CAD build for the part. Positions are in the model's coordinates, mm. A direction names the side the tool comes from. Round coordinates to 2 decimals unless told otherwise and drop trailing zeros. Order: outer loops, then holes, each group sorted by start corner. A loop starts at its lowest first (then second) coordinate and runs counter-clockwise, first axis right, second up. Notation, with made-up numbers: M 51,61.25 L 90,61.25 A18 ccw 90,80.25 Z; hole C 77.25,-30 d10. An arc over 180 degrees is marked long. Put each result on its own line as item: value.
```python
from build123d import *

# Parameters (mm, degrees)
BOSS_EXTRUDE1_DEPTH            = 5
SKETCH2_W                      = 135
SKETCH2_H                      = 160
SKETCH2_W_2                    = 125
SKETCH2_H_2                    = 150
BOSS_EXTRUDE2_DEPTH            = 23
SKETCH3_R                      = 4.7
CUT_EXTRUDE1_DEPTH             = 140
SKETCH4_R                      = 4
BOSS_EXTRUDE3_DEPTH            = 47
F_2_5MM_DOWEL_HOLE1_D          = 2.5
F_2_5MM_DOWEL_HOLE1_DEPTH      = 12
F_2_5MM_DOWEL_HOLE1_TIP        = 0.751075774
FILLET1_R                      = 1
SKETCH8_R                      = 2.5
BOSS_EXTRUDE4_DEPTH            = 4
F_2_5_2_5_DIAMETER_HOLE2_D     = 2.5
F_2_5_2_5_DIAMETER_HOLE2_DEPTH = 5
F_2_5_2_5_DIAMETER_HOLE2_TIP   = 0.751075774
FILLET2_R                      = 10


with BuildPart() as part:
    # Sketch1 → Boss-Extrude1 (new body)
    with BuildSketch(Plane(origin=(0, 0, 0), x_dir=(1, 0, 0), z_dir=(0, 1, 0))):
        with BuildLine():
            Line((-67.5, 80), (-67.5, -80))
            Line((-67.5, -80), (67.5, -80))
            Line((67.5, -80), (67.5, 80))
            Line((67.5, 80), (26.490666647, 192.672217375))
            ThreePointArc((26.490666647, 192.672217375), (0, 211.221181853), (-26.490666647, 192.672217375))
            Line((-26.490666647, 192.672217375), (-67.5, 80))
        make_face()
        Polygon((-37.5, 80), (37.5, 80), (0, 183.03040323), align=None, mode=Mode.SUBTRACT)
    extrude(amount=BOSS_EXTRUDE1_DEPTH)

    # Sketch2 → Boss-Extrude2 (add)
    with BuildSketch(Plane(origin=(0, 5, 0), x_dir=(1, 0, 0), z_dir=(0, 1, 0))):
        Rectangle(SKETCH2_W, SKETCH2_H)
        Rectangle(SKETCH2_W_2, SKETCH2_H_2, mode=Mode.SUBTRACT)
    extrude(amount=BOSS_EXTRUDE2_DEPTH)

    # Sketch3 → Cut-Extrude1 (cut)
    with BuildSketch(Plane(origin=(67.5, 0, 0), x_dir=(0, 0, -1), z_dir=(1, 0, 0))):
        with Locations((-45, 28)):
            Circle(SKETCH3_R)
    extrude(amount=-CUT_EXTRUDE1_DEPTH, mode=Mode.SUBTRACT)

    # Sketch4 → Boss-Extrude3 (add)
    with BuildSketch(Plane(origin=(0, 5, 0), x_dir=(1, 0, 0), z_dir=(0, 1, 0))):
        with Locations(Location((-52.5, 65, 0), (0, 0, 90))):
            Circle(SKETCH4_R)
        with Locations(Location((52.5, 65, 0), (0, 0, 90))):
            Circle(SKETCH4_R)
        with Locations(Location((52.5, -65, 0), (0, 0, 90))):
            Circle(SKETCH4_R)
        with Locations(Location((-52.5, -65, 0), (0, 0, 90))):
            Circle(SKETCH4_R)
    extrude(amount=BOSS_EXTRUDE3_DEPTH)

    # Ø2.5mm Dowel Hole1
    with Locations(Plane(origin=(0, 52, 0), x_dir=(1, 0, 0), z_dir=(0, 1, 0))):
        with Locations((-52.5, 65), (52.5, 65), (52.5, -65), (-52.5, -45), (-52.5, -65)):
            Hole(F_2_5MM_DOWEL_HOLE1_D / 2, depth=F_2_5MM_DOWEL_HOLE1_DEPTH)
            with Locations((0, 0, -(F_2_5MM_DOWEL_HOLE1_DEPTH + F_2_5MM_DOWEL_HOLE1_TIP / 2))):  # 118° drill point
                Cone(0, F_2_5MM_DOWEL_HOLE1_D / 2, F_2_5MM_DOWEL_HOLE1_TIP, mode=Mode.SUBTRACT)

    # Fillet1
    fillet1_edges = [part.edges().sort_by_distance(p)[0] for p in [
        (67.5, 14, 80),
        (-67.5, 14, 80),
        (0, 2.5, -183.03040323),
        (0, 0, 80),
        (-67.5, 0, 0),
        (67.5, 0, 0),
    ]]
    fillet(fillet1_edges, radius=FILLET1_R)

    # Sketch8 → Boss-Extrude4 (add)
    with BuildSketch(Plane(origin=(0, 5, 0), x_dir=(1, 0, 0), z_dir=(0, 1, 0))):
        with Locations(Location((-40.82, 15.565, 0), (0, 0, 90))):
            Circle(SKETCH8_R)
        with Locations(Location((-40.82, -15.565, 0), (0, 0, 90))):
            Circle(SKETCH8_R)
        with Locations(Location((40.82, -15.565, 0), (0, 0, 90))):
            Circle(SKETCH8_R)
        with Locations(Location((40.82, 15.565, 0), (0, 0, 90))):
            Circle(SKETCH8_R)
    extrude(amount=BOSS_EXTRUDE4_DEPTH)

    # Ø2.5 (2.5) Diameter Hole2
    with Locations(Plane(origin=(0, 9, 0), x_dir=(1, 0, 0), z_dir=(0, 1, 0))):
        with Locations((-40.82, 15.565), (-40.82, -15.565), (40.82, -15.565), (40.82, 15.565)):
            Hole(F_2_5_2_5_DIAMETER_HOLE2_D / 2, depth=F_2_5_2_5_DIAMETER_HOLE2_DEPTH)
            with Locations((0, 0, -(F_2_5_2_5_DIAMETER_HOLE2_DEPTH + F_2_5_2_5_DIAMETER_HOLE2_TIP / 2))):  # 118° drill point
                Cone(0, F_2_5_2_5_DIAMETER_HOLE2_D / 2, F_2_5_2_5_DIAMETER_HOLE2_TIP, mode=Mode.SUBTRACT)

    # Fillet2
    fillet2_edges = [part.edges().sort_by_distance(p)[0] for p in [
        (-52.5, 5, -80),
        (52.5, 5, -80),
    ]]
    fillet(fillet2_edges, radius=FILLET2_R)


solid = part.part
```
Item 1: Mould opens along X. For faces 3 (the flat face through (-46.9, 3, -136.6)), 4 (the flat face through (-1, 14, 80)), 5 (the flat face through (62.5, 16, 1)) say: pulls with the +X half, pulls with the -X half, needs draft (parallel to the pull), parting line crosses it, or undercut.
Answers below:
face 3: pulls with the -X half
face 4: needs draft
face 5: undercut
Item 2: Band-saw the part on B-B on x = -6.5. Give the cut face in (y, z).
Answers below:
outline: M 0,-210.46 L 5,-210.46 L 5,-165.17 L 0,-165.17 Z; M 0,-80 L 28,-80 L 28,-75 L 5,-75 L 5,75 L 28,75 L 28,80 L 1,80 A1 ccw 0,79 Z
Item 3: Tool access for faces 1 (the flat face through (41, 9, -14)), 2 (the cylindrical face through (-65, 23.3, 45.1)): list every direction of +Z, -Z, +X, -X, +Y, -Y with a clear straight run to the whole face (end or side of a thin tool).
Answers below:
face 1: +Y
face 2: +X, -X, +Y
Item 4: Band-saw the part on C-C on y = 31. Give the cut face in (x, z).
Answers below:
outline: C -52.5,-65 d8; C -52.5,65 d8; C 52.5,-65 d8; C 52.5,65 d8
Item 5: Band-saw the part on A-A on y = 49. Give the cut face in (x, z), and give its area (3 significant figures).
Answers below:
outline: C -52.5,-65 d8; C -52.5,65 d8; C 52.5,-65 d8; C 52.5,65 d8; hole C -52.5,-65 d2.5; hole C -52.5,65 d2.5; hole C 52.5,-65 d2.5; hole C 52.5,65 d2.5
area: 181 mm²
Item 6: Pin check, flat tips, straight feed: P1, Ø18.5, axis at x = 28.5, y = 19, coming from the -Z side; P2, Ø2.5, axis at x = 42, z = 16.5, coming from the +Y side; P3, Ø2, axis at x = 29, z = -149, coming from the +Y side. Stop position of each tip, or through.
Answers below:
P1: z = -80
P2: y = 9
P3: y = 5
Item 7: Band-saw the part on D-D on z = -158. Give the cut face in (x, y).
Answers below:
outline: M -39.11,0 L -9.11,0 L -9.11,5 L -39.11,5 Z; M 9.11,0 L 39.11,0 L 39.11,5 L 9.11,5 Z
Item 8: Probe line 1 along X through (y, z) = (10, -72.5); line 2 along Z through (x, y) = (52.5, 43.75); line 3 along X through (y, z) = (21, 65). List the from-to ranges inside material, lowest first. Write a range as [from, to].
Answers below:
line 1: [-67.5, -62.5], [62.5, 67.5]
line 2: [-69, -66.25], [-63.75, -61], [61, 63.75], [66.25, 69]
line 3: [-67.5, -62.5], [-56.5, -48.5], [48.5, 56.5], [62.5, 67.5]
